```python
from build123d import *

# Parameters (mm, degrees)
F1_DEPTH = 6
F3_DEPTH = 10


with BuildPart() as f1:
    # F0 (on Top) → F1 (new body, symmetric)
    with BuildSketch(Plane.XY):
        with BuildLine():
            Line((6.5, -5.25), (6.5, 5.25))
            ThreePointArc((6.5, 5.25), (6.133883, 6.133883), (5.25, 6.5))
            Line((5.25, 6.5), (-5.25, 6.5))
            ThreePointArc((-5.25, 6.5), (-6.133883, 6.133883), (-6.5, 5.25))
            Line((-6.5, 5.25), (-6.5, -5.25))
            ThreePointArc((-6.5, -5.25), (-6.133883, -6.133883), (-5.25, -6.5))
            Line((-5.25, -6.5), (5.25, -6.5))
            ThreePointArc((5.25, -6.5), (6.133883, -6.133883), (6.5, -5.25))
        make_face()
    extrude(amount=F1_DEPTH, both=True)

    # F2 (on Top) → F3 (cut, symmetric)
    with BuildSketch(Plane.XY):
        with BuildLine():
            ThreePointArc((0.889914, -2.1566), (0.928239, -2.163918), (0.961171, -2.184843))
            Line((0.961171, -2.184843), (2.745753, -3.863205))
            Line((2.745753, -3.863205), (1.752595, -3.863205))
            ThreePointArc((1.752595, -3.863205), (1.466924, -3.981534), (1.348595, -4.267205))
            Line((1.348595, -4.267205), (1.348595, -4.749805))
            ThreePointArc((1.348595, -4.749805), (1.466924, -5.035476), (1.752595, -5.153805))
            Line((1.752595, -5.153805), (4.749795, -5.153805))
            ThreePointArc((4.749795, -5.153805), (5.035466, -5.035476), (5.153795, -4.749805))
            Line((5.153795, -4.749805), (5.153795, -1.752605))
            ThreePointArc((5.153795, -1.752605), (5.035471, -1.466932), (4.749802, -1.348599))
            Line((4.749802, -1.348599), (4.267202, -1.348599))
            ThreePointArc((4.267202, -1.348599), (3.981531, -1.466927), (3.863202, -1.752599))
            Line((3.863202, -1.752599), (3.863202, -2.745756))
            Line((3.863202, -2.745756), (2.184831, -0.961164))
            ThreePointArc((2.184831, -0.961164), (2.163912, -0.928237), (2.156595, -0.889919))
            Line((2.156595, -0.889919), (2.156595, 0.889909))
            ThreePointArc((2.156595, 0.889909), (2.163912, 0.928229), (2.184834, 0.961157))
            Line((2.184834, 0.961157), (3.863202, 2.745746))
            Line((3.863202, 2.745746), (3.863202, 1.752589))
            ThreePointArc((3.863202, 1.752589), (3.981531, 1.466917), (4.267202, 1.348589))
            Line((4.267202, 1.348589), (4.749802, 1.348589))
            ThreePointArc((4.749802, 1.348589), (5.035473, 1.466917), (5.153802, 1.752589))
            Line((5.153802, 1.752589), (5.153802, 4.749789))
            ThreePointArc((5.153802, 4.749789), (5.035477, 5.035475), (4.749794, 5.153807))
            Line((4.749794, 5.153807), (1.752594, 5.153807))
            ThreePointArc((1.752594, 5.153807), (1.466922, 5.035478), (1.348594, 4.749807))
            Line((1.348594, 4.749807), (1.348594, 4.267207))
            ThreePointArc((1.348594, 4.267207), (1.466922, 3.981536), (1.752594, 3.863207))
            Line((1.752594, 3.863207), (2.745751, 3.863207))
            Line((2.745751, 3.863207), (0.961159, 2.184836))
            ThreePointArc((0.961159, 2.184836), (0.928232, 2.163916), (0.889914, 2.1566))
            Line((0.889914, 2.1566), (-0.889914, 2.1566))
            ThreePointArc((-0.889914, 2.1566), (-0.928238, 2.163918), (-0.961169, 2.184841))
            Line((-0.961169, 2.184841), (-2.745757, 3.863209))
            Line((-2.745757, 3.863209), (-1.7526, 3.863209))
            ThreePointArc((-1.7526, 3.863209), (-1.466929, 3.981538), (-1.3486, 4.267209))
            Line((-1.3486, 4.267209), (-1.3486, 4.749809))
            ThreePointArc((-1.3486, 4.749809), (-1.466937, 5.035473), (-1.752607, 5.153794))
            Line((-1.752607, 5.153794), (-4.749807, 5.153794))
            ThreePointArc((-4.749807, 5.153794), (-5.035478, 5.035465), (-5.153807, 4.749794))
            Line((-5.153807, 4.749794), (-5.153807, 1.752594))
            ThreePointArc((-5.153807, 1.752594), (-5.035478, 1.466922), (-4.749807, 1.348594))
            Line((-4.749807, 1.348594), (-4.267207, 1.348594))
            ThreePointArc((-4.267207, 1.348594), (-3.981536, 1.466922), (-3.863207, 1.752594))
            Line((-3.863207, 1.752594), (-3.863207, 2.745751))
            Line((-3.863207, 2.745751), (-2.184836, 0.961159))
            ThreePointArc((-2.184836, 0.961159), (-2.163916, 0.928232), (-2.1566, 0.889914))
            Line((-2.1566, 0.889914), (-2.1566, -0.889914))
            ThreePointArc((-2.1566, -0.889914), (-2.163918, -0.928238), (-2.184841, -0.961169))
            Line((-2.184841, -0.961169), (-3.863209, -2.745757))
            Line((-3.863209, -2.745757), (-3.863209, -1.7526))
            ThreePointArc((-3.863209, -1.7526), (-3.981538, -1.466929), (-4.267209, -1.3486))
            Line((-4.267209, -1.3486), (-4.749809, -1.3486))
            ThreePointArc((-4.749809, -1.3486), (-5.035481, -1.466929), (-5.153809, -1.7526))
            Line((-5.153809, -1.7526), (-5.153809, -4.7498))
            ThreePointArc((-5.153809, -4.7498), (-5.035481, -5.035471), (-4.749809, -5.1538))
            Line((-4.749809, -5.1538), (-1.752609, -5.1538))
            ThreePointArc((-1.752609, -5.1538), (-1.466938, -5.035471), (-1.348609, -4.7498))
            Line((-1.348609, -4.7498), (-1.348609, -4.2672))
            ThreePointArc((-1.348609, -4.2672), (-1.466935, -3.981539), (-1.752594, -3.863207))
            Line((-1.752594, -3.863207), (-2.745751, -3.863207))
            Line((-2.745751, -3.863207), (-0.961159, -2.184836))
            ThreePointArc((-0.961159, -2.184836), (-0.928232, -2.163916), (-0.889914, -2.1566))
            Line((-0.889914, -2.1566), (0.889914, -2.1566))
        make_face()
    extrude(amount=F3_DEPTH, both=True, mode=Mode.SUBTRACT)


solid = f1.part
```
Build history of the part. All positions in model axes, mm. A direction names the side the tool comes from. Round coordinates to 2 decimals unless told otherwise and drop trailing zeros. Write each loop counter-clockwise with the first axis right and the second up, starting at its lowest first coordinate (ties: lowest second). Pieces come first, ordered by that corner, then holes.
1) Mould opens along Y. For faces 3 (the flat face through (-3, -5.154, 0)), 4 (the cylindrical face through (6.144, 6.124, 0.084)), 5 (the flat face through (2, -3.863, 0)), 6 (the cylindrical face through (6.124, -6.144, 0.084)) say: +Y half, -Y half, draft (parallel to the pull), parting line (faces both ways), or undercut.
2) Band-saw the part on B-B, the plane y = 3.5. List the corners of the cut face in (x, z), and give its area (3 significant figures).
3) Drill centre lines: probe 1 along Y at (x, z) = (4.25, 0.5); probe 2 along Y at (x, z) = (-0.75, 3). Where is each one in solid material? Low to high.
4) 3-axis set-ups, long thin cutter, end or side, ignore diameter. For faces 1 (the flat face through (6.5, 0, 0)), 2 (the flat face through (-2.157, 0, 0)): which of +Z, -Z, +X, -X, +Y, -Y reach the whole face in a straight line?
5) Band-saw the part on A-A, the plane x = -3. List the corners of the cut face in (y, z), and give its area (3 significant figures).
Ans:
1. face 3: undercut
1. face 4: +Y half
1. face 5: undercut
1. face 6: -Y half
2. outline: (-6.5, -6) - (-5.15, -6) - (-5.15, 6) - (-6.5, 6) - close; (-2.36, -6) - (2.36, -6) - (2.36, 6) - (-2.36, 6) - close; (5.15, -6) - (6.5, -6) - (6.5, 6) - (5.15, 6) - close
2. area: 88.9 mm2
3. probe 1: y = -6.5 to -5.15, -1.35 to 1.35, 5.15 to 6.5
3. probe 2: y = -6.5 to -2.16, 2.16 to 6.5
4. face 1: +Z, -Z, +X, +Y, -Y
4. face 2: +Z, -Z
5. outline: (-6.5, -6) - (-5.15, -6) - (-5.15, 6) - (-6.5, 6) - close; (-1.83, -6) - (1.83, -6) - (1.83, 6) - (-1.83, 6) - close; (5.15, -6) - (6.5, -6) - (6.5, 6) - (5.15, 6) - close
5. area: 76.2 mm2
